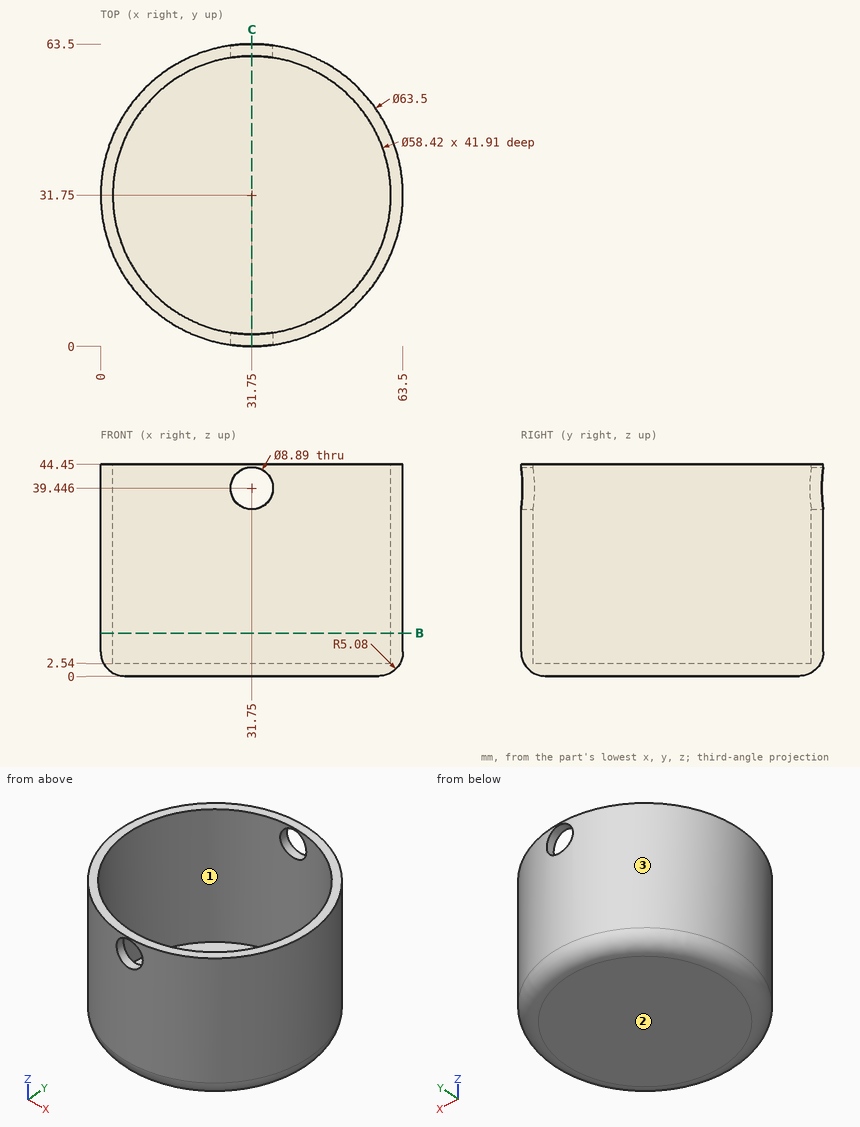
Here's the drawing with two shaded views (mm, measured from the low corner). I have some questions. Give positions to 0.01 mm unless a question says otherwise; leave off trailing zeros. Write each loop counter-clockwise with the first axis right and the second up, starting at its lowest first coordinate (ties: lowest second). Pieces come first, ordered by that corner, then holes. Notation, with made-up numbers: (62.25, 50) - (70.25, 50) arc R20 cw to (70.25, 58) - close; hole circle Ø11 at (36.25, 47.5). An arc over 180 degrees is marked (long way). One line per item, written item: value. Start each with the question number.
Item 1: Imagine slicing it at B-B, the plane z = 9. List the corners of the cut face in (x, y) for me.
Item 2: Imagine slicing it at C-C, the plane x = 31.75. Give the number of separate pieces and of enclosed holes in the cut face, and give its area (3 significant figures).
Item 3: If we mould it in two halves opening along X, with no side actions, what happens to the marked faces 1, 2 and 3? For each: +X half, -X half, draft (parallel to the pull), parting line (faces both ways), or undercut.
Item 4: I'm going to push flat-ended pins straight in: pin 1 (2 mm diameter, centred on x = 29, z = 9, fed in from -Y); pin 2 (17.5 mm diameter, centred on x = 45, y = 24.5, fed in from +Z); pin 3 (6 mm diameter, centred on y = 18, z = 20.5, fed in from +X) (1 decimal). Where does each tip first touch, or does it pass through?
Item 5: Please list where these lines run through material, in increasing order: line 1 (X direction, y = 31, z = 12); line 2 (Y direction, x = 32, z = 9). Write a range as from..to.
Geometry says:
1. outline: circle Ø63.5 at (31.75, 31.75); hole circle Ø58.42 at (31.75, 31.75)
2. separate pieces: 3
2. enclosed holes: 0
2. area: 318 mm^2
3. face 1: undercut
3. face 2: draft
3. face 3: parting line
4. pin 1: y = 0.05
4. pin 2: z = 2.54
4. pin 3: x = 61.6
5. line 1: 0.01..2.55, 60.95..63.49
5. line 2: 0..2.54, 60.96..63.5
